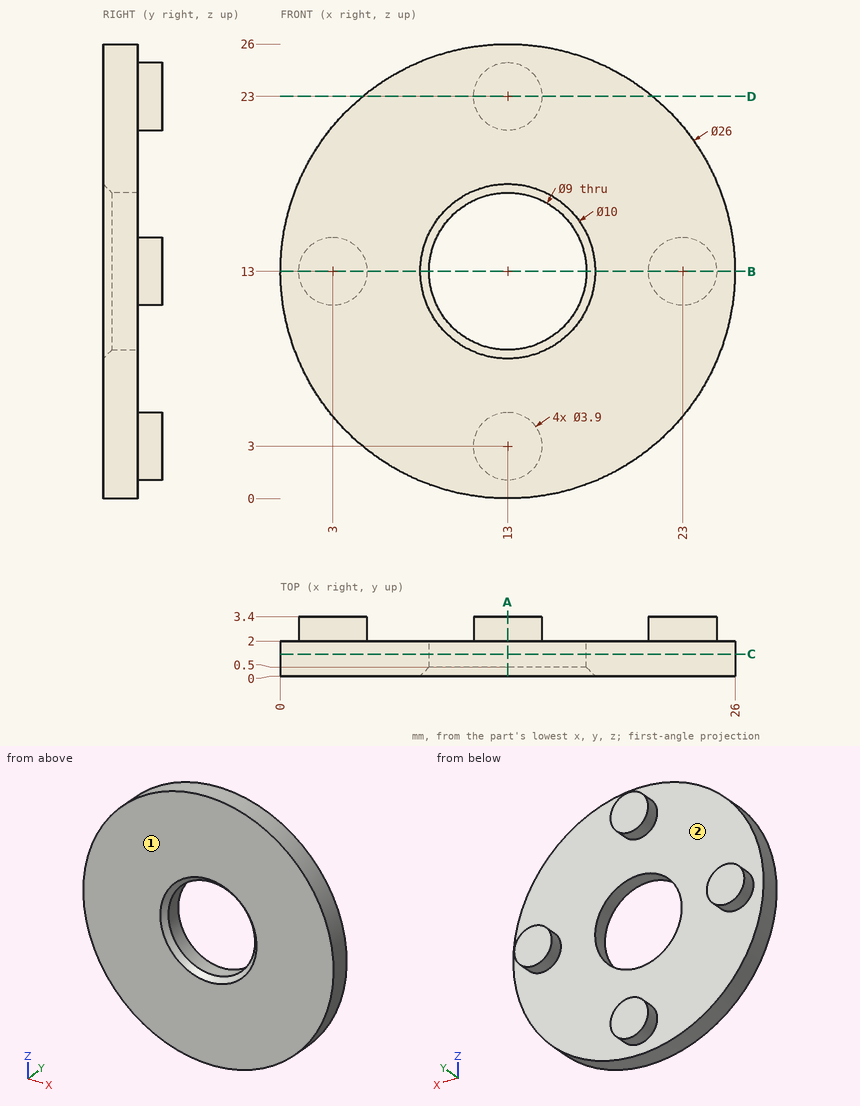
Drawing for the job (mm, zero at the part's lowest x, y, z). A direction names the side the tool comes from. Give positions to 0.01 mm unless a question says otherwise; leave off trailing zeros. Order: outer loops, then holes, each group sorted by start corner. A loop starts at its lowest first (then second) coordinate and runs counter-clockwise, first axis right, second up. Notation, with made-up numbers: M 54.25,70.25 L 99.25,70.25 A34 ccw 99.25,108.25 Z; hole C 62.25,-16 d11. An arc over 180 degrees is marked long. Use a Markdown table: item, result. Add a question column.
(1) 3-axis set-ups, long thin cutter, end or side, ignore diameter. For the marked faces 1 and 2: which of +Z, -Z, +X, -X, +Y, -Y reach the whole face in a straight line?
(2) Saw through at C-C, the plane y = 1.25. Give the cut face in (x, z).
(3) Saw through at A-A, the plane x = 13. Give the cut face in (y, z), and give its area (3 significant figures).
(4) Saw through at B-B, the plane z = 13. Give the cut face in (x, y), and give its area (3 significant figures).
(5) Probe line 1 along X through (y, z) = (0.9, 13); line 2 along Y through (x, z) = (8.75, 21); line 3 along Z through (x, y) = (14, 1.3). List the from-to ranges inside material, lowest first. Write a range as [from, to].
(6) Saw through at D-D, the plane z = 23. Give the cut face in (x, y), and give its area (3 significant figures).
(7) Drop flat-ended pins along their axis: P1, Ø8, axis at x = 16, z = 16, coming from the -Y side; P2, Ø5, axis at x = 13, z = 10, coming from the +Y side; P3, Ø1.5, axis at y = 1, z = 23, coming from the -X side. Give the stop position or say it passes through.
Answer key:
| question | item | result |
|---|---|---|
| 1 | face 1 | +Z, -Z, +X, -X, -Y |
| 1 | face 2 | +Y |
| 2 | outline | C 13,13 d26; hole C 13,13 d9 |
| 3 | outline | M 0,0 L 2,0 L 2,1.05 L 3.4,1.05 L 3.4,4.95 L 2,4.95 L 2,8.5 L 0.5,8.5 L 0,8 Z; M 0,18 L 0.5,17.5 L 2,17.5 L 2,21.05 L 3.4,21.05 L 3.4,24.95 L 2,24.95 L 2,26 L 0,26 Z |
| 3 | area | 44.7 mm^2 |
| 4 | outline | M 0,0 L 8,0 L 8.5,0.5 L 8.5,2 L 4.95,2 L 4.95,3.4 L 1.05,3.4 L 1.05,2 L 0,2 Z; M 17.5,0.5 L 18,0 L 26,0 L 26,2 L 24.95,2 L 24.95,3.4 L 21.05,3.4 L 21.05,2 L 17.5,2 Z |
| 4 | area | 44.7 mm^2 |
| 5 | line 1 | [0, 8.5], [17.5, 26] |
| 5 | line 2 | [0, 2] |
| 5 | line 3 | [0.04, 8.61], [17.39, 25.96] |
| 6 | outline | M 4.69,0 L 21.31,0 L 21.31,2 L 14.95,2 L 14.95,3.4 L 11.05,3.4 L 11.05,2 L 4.69,2 Z |
| 6 | area | 38.7 mm^2 |
| 7 | P1 | y = 0 |
| 7 | P2 | y = 2 |
| 7 | P3 | x = 3.87 |
